from build123d import *

# Parameters (mm, degrees)
CUT_EXTRUDE1_DEPTH = 2.08359375
CHAMFER1_SIZE      = 0.28702
CHAMFER2_SIZE      = 0.14351


with BuildPart() as part:
    # Sketch2 → Revolve1 (revolve)
    with BuildSketch(Plane(origin=(0, 0, 0), x_dir=(0, 0, -1), z_dir=(1, 0, 0)), mode=Mode.PRIVATE) as revolve1_sk:
        Polygon((8.1026, 1.1572875), (7.5072875, 1.7526), (-4.5974, 1.7526), (-4.5974, 2.8702), (-8.1026, 2.8702), (-8.1026, 0), (8.1026, 0), align=None)
    revolve(revolve1_sk.sketch.rotate(Axis((0, 0, -8.1026), (0, 0, 1)), 90), axis=Axis((0, 0, -8.1026), (0, 0, 1)))

    # Sketch4 → Cut-Extrude1 (cut)
    with BuildSketch(Plane.XY.offset(8.1026)):
        Polygon((0, 1.603951217), (-1.3890625, 0.801975608), (-1.3890625, -0.801975608), (0, -1.603951217), (1.3890625, -0.801975608), (1.3890625, 0.801975608), align=None)
    extrude(amount=-CUT_EXTRUDE1_DEPTH, mode=Mode.SUBTRACT)

    # Cut-Extrude2 cone 1 section (on through the dimple's axis) → Cut-Extrude2 (revolve, cut)
    with BuildSketch(Plane(origin=(0, 0, 8.1026), x_dir=(0, -1, 0), z_dir=(1, 0, 0))):
        Polygon((0, 0), (1.603951217, 0), (0, 0.926041667), align=None)
    revolve(axis=Axis((0, 0, 8.1026), (0, 0, -1)), mode=Mode.SUBTRACT)

    # Chamfer1
    chamfer1_edges = [part.edges().sort_by_distance(p)[0] for p in [
        (2.8702, 0, 8.1026),
    ]]
    chamfer(chamfer1_edges, length=CHAMFER1_SIZE)

    # Chamfer2
    chamfer2_edges = [part.edges().sort_by_distance(p)[0] for p in [
        (2.8702, 0, 4.5974),
    ]]
    chamfer(chamfer2_edges, length=CHAMFER2_SIZE)


solid = part.part
For this review, take the finished solid that the model builds, in its own axes (mm). A direction names the side the tool comes from. Round coordinates to 2 decimals unless told otherwise and drop trailing zeros. Write each loop counter-clockwise with the first axis right and the second up, starting at its lowest first coordinate (ties: lowest second). Pieces come first, ordered by that corner, then holes. Notation, with made-up numbers: (68, -26.75) -> (92, -26.75) arc R6 ccw to (92, -22.75) -> close; hole circle Ø9 at (61.5, -23). An arc over 180 degrees is marked (long way). Use CSV: the item, a comma, the result in double quotes.
(1) Consider section B-B, the plane z = -2. Give the boundary of the cut face in (x, y), plus the area to 3 significant figures.
Computed values:
outline,"circle Ø3.51 at (0, 0)"
area,"9.65 mm²"
(2) For faces 1 (the face through (-2.74, -0.86, 6.3)), 2 (the face through (-0.7, -1.2, 7.1)), list the 3-axis set-ups (+Z, -Z, +X, -X, +Y, -Y) from which the entire face can be reached by the end or side of a thin tool; tool diameter is ignored.
Computed values:
face 1,"+Z, -Z"
face 2,"+Z"
(3) Clearance check with flat-ended pins moving along their axes: P1, Ø3, axis at y = -2.5, z = 0, coming from the -X side; P2, Ø2, axis at y = 1.5, z = -4.5, coming from the -X side; P3, Ø1.5, axis at x = -1.5, y = 1.5, coming from the -Z side. State where each tip first meets the part, or that it passes through.
Computed values:
P1,"x = -1.44"
P2,"x = -1.68"
P3,"z = -7.89"
(4) Consider section A-A, the plane y = 0. Give the boundary of the cut face in (x, z), plus the area to 3 significant figures.
Computed values:
outline,"(-2.87, 4.74) -> (-2.73, 4.6) -> (-1.75, 4.6) -> (-1.75, -7.51) -> (-1.16, -8.1) -> (1.16, -8.1) -> (1.75, -7.51) -> (1.75, 4.6) -> (2.73, 4.6) -> (2.87, 4.74) -> (2.87, 7.82) -> (2.58, 8.1) -> (1.6, 8.1) -> (1.39, 7.98) -> (1.39, 6.02) -> (-1.39, 6.02) -> (-1.39, 7.98) -> (-1.6, 8.1) -> (-2.58, 8.1) -> (-2.87, 7.82) -> close"
area,"58.4 mm²"
(5) To check wall thickness, follow L1, parallel to Z at x = -0.8, y = 1.7; L2, parallel to Z at x = 0, y = 1.1; L3, parallel to X at y = 0.7, z = -6.25. State the ranges of each line that lie inside material, in increasing order. Write a range as [from, to].
Computed values:
L1,"[4.6, 8.1]"
L2,"[-8.1, 6.02]"
L3,"[-1.61, 1.61]"
(6) Draft analysis for pull direction Y (two halves, no side actions). For faces 3 (the face through (0, 2, 4.597)), 4 (the face through (-1.67, -0.53, -1.37)), 5 (the face through (1.389, 0, 7)), state which applies: +Y half, -Y half, draft (parallel to the pull), parting line (faces both ways), or undercut.
Computed values:
face 3,"draft"
face 4,"parting line"
face 5,"undercut"
